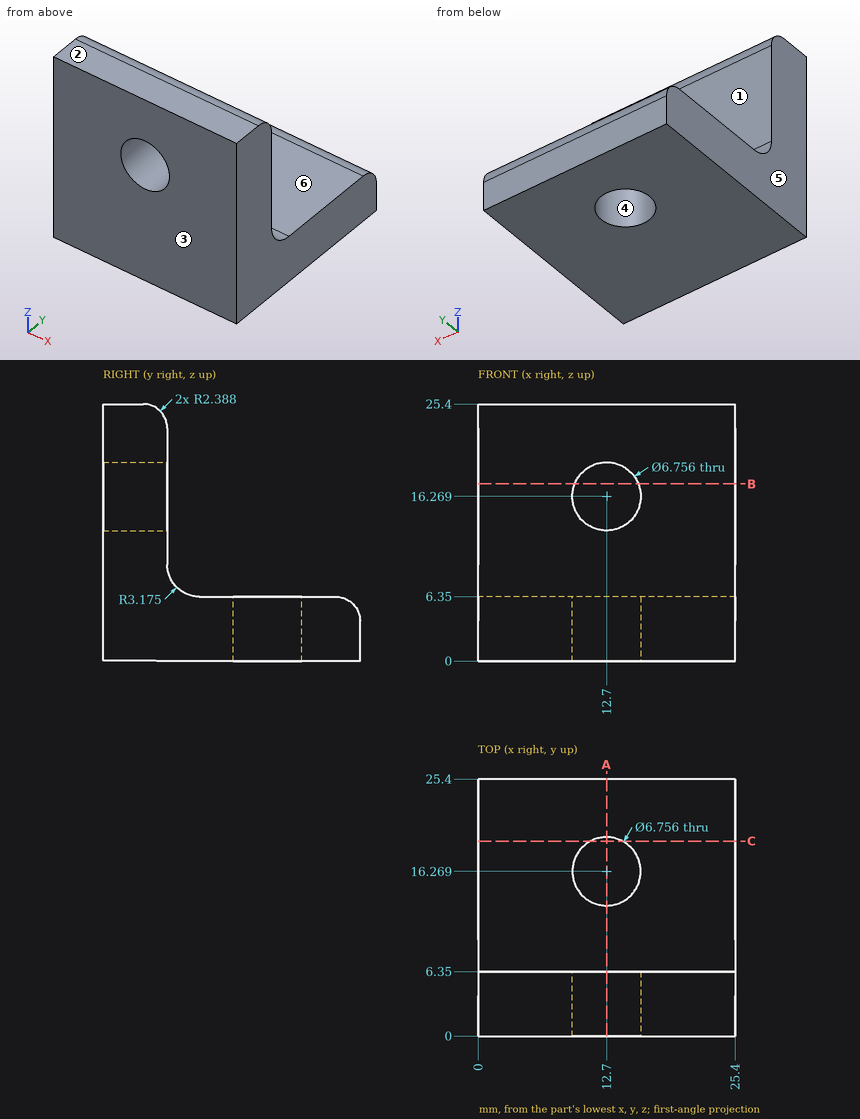
Check sheet for the drawn part. Datum: minimum x, y, z corner. Units: mm. A direction names the side the tool comes from. Round coordinates to 2 decimals unless told otherwise and drop trailing zeros. Order: outer loops, then holes, each group sorted by start corner. A loop starts at its lowest first (then second) coordinate and runs counter-clockwise, first axis right, second up.
1) Section check C-C (y = 19.25). Record the boundary of the cut face in (x, z), and give its area (3 significant figures).
2) Section check B-B (z = 17.5). Record the boundary of the cut face in (x, y), and give its area (3 significant figures).
3) Section check A-A (x = 12.7). Give the number of separate pieces and of enclosed holes in the cut face, and give its area (3 significant figures).
4) Scan lines: line 1 (Y direction, x = 12.7, z = 3.75); line 2 (Z direction, x = 10.25, y = 12). Record each from-to range of solid material in increasing order.
5) Go/stop test with flat-tipped pins: pin 1 Ø1.5 at (x, y) = (5.5, 11) entering from +Z; pin 2 Ø9 at (x, y) = (12.7, 16.27) entering from -Z; pin 3 Ø8 at (x, z) = (12.7, 16.27) entering from +Y; pin 4 Ø1.5 at (x, z) = (13, 6.5) entering from +Y (1 decimal). Record where each tip stops, or that it passes through.
6) Mould release check, pull along Y, two halves, no side actions. Record for the marked faces 1, 2, 3 and 4: +Y half, -Y half, draft (parallel to the pull), parting line (faces both ways), or undercut.
7) Tool access check on the marked faces 5 and 6. Record the directions out of +Z, -Z, +X, -X, +Y, -Y that give a thin tool (end or side, any length) a straight path to the whole face; none if there is none.
Result:
1. outline: (0, 0) - (11.11, 0) - (11.11, 6.35) - (0, 6.35) - close; (14.29, 0) - (25.4, 0) - (25.4, 6.35) - (14.29, 6.35) - close
1. area: 141 mm2
2. outline: (0, 0) - (9.55, 0) - (9.55, 6.35) - (0, 6.35) - close; (15.85, 0) - (25.4, 0) - (25.4, 6.35) - (15.85, 6.35) - close
2. area: 121 mm2
3. separate pieces: 3
3. enclosed holes: 0
3. area: 196 mm2
4. line 1: y = 0 to 12.89, 19.65 to 25.4
4. line 2: z = 0 to 6.35
5. pin 1: stops at z = 6.35
5. pin 2: stops at z = 0
5. pin 3: stops at y = 6.35
5. pin 4: stops at y = 24.6
6. face 1: +Y half
6. face 2: draft
6. face 3: -Y half
6. face 4: undercut
7. face 5: +Z, -Z, -X, +Y, -Y
7. face 6: +Z, +X, -X, +Y
